Could you check a few things on this model? Use its own coordinates, in mm. Face numbers are marked on the shaded views. A direction names the side the tool comes from. Give positions to 0.01 mm unless a question says otherwise; leave off trailing zeros. Order: outer loops, then holes, each group sorted by start corner. A loop starts at its lowest first (then second) coordinate and runs counter-clockwise, first axis right, second up. Notation, with made-up numbers: M 17.25,42 L 76.25,42 A19 cw 76.25,65 Z; hole C -33,75.5 d9. An arc over 180 degrees is marked long. Use a Markdown table: item, result. Add a question column.
Item 1: Suppose I cut it at C-C on y = -49.5. Write out the boundary of the cut face in (x, z), plus the area to 3 significant figures.
Item 2: Suppose I cut it at D-D on x = 0. Write out the boundary of the cut face in (y, z).
Item 3: I'm going to push flat-ended pins straight in: pin 1 Ø2 at (x, z) = (2.5, -9.5) entering from +Y; pin 2 Ø3 at (x, y) = (30, -49.5) entering from +Z; pin 3 Ø1.5 at (x, z) = (46, -10) entering from -Y. Where does each tip first touch, or does it pass through?
Item 4: If I drill on L1, parallel to X at y = 3.3, z = -15.5; L2, parallel to Z at x = 23.5, y = -11; L3, parallel to X at y = -25.5, z = -3, over which ranges is the centre line in solid material (lowest first)? Write a range as from..to.
Item 5: If we mould it in two halves opening along X, with no side actions, what happens to the marked faces 4, 5 and 6? For each: released by +X, released by -X, zero draft, split by the parting line, or undercut.
Item 6: Suppose I cut it at B-B on x = -30. Write out the boundary of the cut face in (y, z), plus the area to 4 significant figures.
Item 7: Suppose I cut it at A-A on z = 15.5. Write out the boundary of the cut face in (x, y).
Item 8: For the marked faces 1, 2 and 3, which set-ups out of +Z, -Z, +X, -X, +Y, -Y let a thin tool reach every point of the face, with its end or its side?
from build123d import *

# Parameters (mm, degrees)
SKETCH_1_W             = 125
SKETCH_1_H             = 55
EXTRUDE_1_DEPTH        = 6
SKETCH_2_R             = 11
CUT_EXTRUDE_1_DEPTH    = 2
CUT_EXTRUDE_2_REACH    = 70.4
SKETCH_3_R             = 2.5
HOLE_WIZARD_M3_1_D     = 2.5
HOLE_WIZARD_M3_1_DEPTH = 7.5
HOLE_WIZARD_M3_1_TIP   = 0.751075774
SKETCH_6_W             = 125
SKETCH_6_H             = 55
SKETCH_6_W_2           = 120
SKETCH_6_H_2           = 50
EXTRUDE_2_DEPTH        = 57
HOLE_WIZARD_M3_2_D     = 2.5
HOLE_WIZARD_M3_2_DEPTH = 2.5
HOLE_WIZARD_M3_3_D     = 2.5


with BuildPart() as part:
    # 草图1 → 凸台-拉伸1 (new body)
    with BuildSketch(Plane(origin=(0, 0, 0), x_dir=(1, 0, 0), z_dir=(0, 1, 0))):
        Rectangle(SKETCH_1_W, SKETCH_1_H)
    extrude(amount=EXTRUDE_1_DEPTH)

    # 草图2 → 切除-拉伸1 (cut)
    with BuildSketch(Plane(origin=(0, 6, 0), x_dir=(1, 0, 0), z_dir=(0, 1, 0))):
        with Locations(Location((0, 0, 0), (0, 0, 270))):
            Circle(SKETCH_2_R)
    extrude(amount=-CUT_EXTRUDE_1_DEPTH, mode=Mode.SUBTRACT)

    # 草图3 → 切除-拉伸2 (cut, up to next)
    with BuildSketch(Plane(origin=(0, 4, 0), x_dir=(1, 0, 0), z_dir=(0, 1, 0)), mode=Mode.PRIVATE) as cut_extrude_2_sk1:
        with Locations(Location((0, 0, 0), (0, 0, 270))):
            Circle(SKETCH_3_R)
    cut_extrude_2_tool1 = extrude(cut_extrude_2_sk1.sketch, amount=-CUT_EXTRUDE_2_REACH, mode=Mode.PRIVATE) & part.part
    add(cut_extrude_2_tool1.solids().sort_by_distance((0, 4, 0))[0], mode=Mode.SUBTRACT)

    # M3 螺纹孔1
    with Locations(Plane(origin=(0, 6, 0), x_dir=(1, 0, 0), z_dir=(0, 1, 0))):
        with Locations((15.5, 15.5), (15.5, -15.5), (-15.5, -15.5), (-15.5, 15.5)):
            Hole(HOLE_WIZARD_M3_1_D / 2, depth=HOLE_WIZARD_M3_1_DEPTH)
            with Locations((0, 0, -(HOLE_WIZARD_M3_1_DEPTH + HOLE_WIZARD_M3_1_TIP / 2))):  # 118° drill point
                Cone(0, HOLE_WIZARD_M3_1_D / 2, HOLE_WIZARD_M3_1_TIP, mode=Mode.SUBTRACT)

    # 草图6 → 凸台-拉伸2 (add)
    with BuildSketch(Plane.XZ):
        Rectangle(SKETCH_6_W, SKETCH_6_H)
        Rectangle(SKETCH_6_W_2, SKETCH_6_H_2, mode=Mode.SUBTRACT)
    extrude(amount=EXTRUDE_2_DEPTH)

    # M3 螺纹孔2
    with Locations(Plane(origin=(0, 0, -27.5), x_dir=(-1, 0, 0), z_dir=(0, 0, -1))):
        with Locations((30, -49.5), (-30, -49.5)):
            Hole(HOLE_WIZARD_M3_2_D / 2, depth=HOLE_WIZARD_M3_2_DEPTH)

    # M3 螺纹孔3 (through all)
    with Locations(Plane.XY.offset(27.5)):
        with Locations((30, -49.5), (-30, -49.5)):
            Hole(HOLE_WIZARD_M3_3_D / 2)


solid = part.part
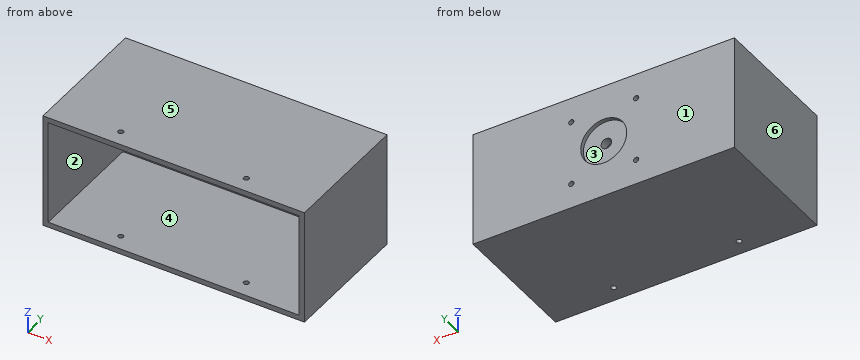
Findings below:
| question | item | result |
|---|---|---|
| 1 | outline | M -62.5,-27.5 L -31.25,-27.5 L -31.25,-25 L -60,-25 L -60,25 L -31.25,25 L -31.25,27.5 L -62.5,27.5 Z; M -28.75,-27.5 L 28.75,-27.5 L 28.75,-25 L -28.75,-25 Z; M -28.75,25 L 28.75,25 L 28.75,27.5 L -28.75,27.5 Z; M 31.25,-27.5 L 62.5,-27.5 L 62.5,27.5 L 31.25,27.5 L 31.25,25 L 60,25 L 60,-25 L 31.25,-25 Z |
| 1 | area | 850 mm^2 |
| 2 | outline | M -57,-27.5 L 6,-27.5 L 6,-11 L 4,-11 L 4,-2.5 L 0,-2.5 L 0,-25 L -57,-25 Z; M -57,25 L 0,25 L 0,2.5 L 4,2.5 L 4,11 L 6,11 L 6,27.5 L -57,27.5 Z |
| 3 | pin 1 | stops at y = 4 |
| 3 | pin 2 | stops at z = 27.5 |
| 3 | pin 3 | stops at y = 0 |
| 4 | L1 | x = -62.5..-16.75, -14.25..14.25, 16.75..62.5 |
| 4 | L2 | z = -27.5..-25, 25..27.5 |
| 4 | L3 | x = -62.5..-60, 60..62.5 |
| 5 | face 4 | undercut |
| 5 | face 5 | zero draft |
| 5 | face 6 | released by -X |
| 6 | outline | M -57,-27.5 L -50.75,-27.5 L -50.75,-25 L -57,-25 Z; M -57,25 L -50.75,25 L -50.75,27.5 L -57,27.5 Z; M -48.25,-27.5 L 6,-27.5 L 6,27.5 L -48.25,27.5 L -48.25,25 L 0,25 L 0,-25 L -48.25,-25 Z |
| 6 | area | 602.5 mm^2 |
| 7 | outline | M -62.5,-57 L -60,-57 L -60,0 L -16.75,0 L -16.75,6 L -62.5,6 Z; M -14.25,0 L 14.25,0 L 14.25,6 L -14.25,6 Z; M 16.75,0 L 60,0 L 60,-57 L 62.5,-57 L 62.5,6 L 16.75,6 Z |
| 8 | face 1 | +Z, -Z, +X, -X, +Y |
| 8 | face 2 | -Y |
| 8 | face 3 | +Y |
